from build123d import *

# Parameters (mm, degrees)
BOSS_EXTRUDE1_DEPTH = 33
SKETCH2_R           = 1
CUT_EXTRUDE1_DEPTH  = 3.5
SKETCH3_W           = 12
SKETCH3_H           = 2
BOSS_EXTRUDE2_DEPTH = 8
SKETCH4_R           = 7.5
BOSS_EXTRUDE3_DEPTH = 1.5
SKETCH5_R           = 2
BOSS_EXTRUDE4_DEPTH = 8.5


with BuildPart() as part:
    # Sketch1 → Boss-Extrude1 (new body)
    with BuildSketch(Plane.XY):
        with BuildLine():
            Line((-8.1, -10.1), (8.1, -10.1))
            ThreePointArc((8.1, -10.1), (9.514213562, -9.514213562), (10.1, -8.1))
            Line((10.1, -8.1), (10.1, 8.1))
            ThreePointArc((10.1, 8.1), (9.514213562, 9.514213562), (8.1, 10.1))
            Line((8.1, 10.1), (-8.1, 10.1))
            ThreePointArc((-8.1, 10.1), (-9.514213562, 9.514213562), (-10.1, 8.1))
            Line((-10.1, 8.1), (-10.1, -8.1))
            ThreePointArc((-10.1, -8.1), (-9.514213562, -9.514213562), (-8.1, -10.1))
        make_face()
    extrude(amount=-BOSS_EXTRUDE1_DEPTH)

    # Sketch2 → Cut-Extrude1 (cut)
    with BuildSketch(Plane.XY):
        with Locations((-8, 8)):
            Circle(SKETCH2_R)
        with Locations((8, 8)):
            Circle(SKETCH2_R)
        with Locations((8, -8)):
            Circle(SKETCH2_R)
        with Locations((-8, -8)):
            Circle(SKETCH2_R)
    extrude(amount=-CUT_EXTRUDE1_DEPTH, mode=Mode.SUBTRACT)

    # Sketch3 → Boss-Extrude2 (add)
    with BuildSketch(Plane(origin=(0, 0, -33), x_dir=(-1, 0, 0), z_dir=(0, 0, -1))):
        with Locations((0, 11.1)):
            Rectangle(SKETCH3_W, SKETCH3_H)
    extrude(amount=-BOSS_EXTRUDE2_DEPTH)

    # Sketch4 → Boss-Extrude3 (add)
    with BuildSketch(Plane.XY):
        with Locations(Location((0, 0, 0), (0, 0, 180))):
            Circle(SKETCH4_R)
    extrude(amount=BOSS_EXTRUDE3_DEPTH)

    # Sketch5 → Boss-Extrude4 (add)
    with BuildSketch(Plane.XY.offset(1.5)):
        Circle(SKETCH5_R)
    extrude(amount=BOSS_EXTRUDE4_DEPTH)


solid = part.part
Build history of the part. All positions in model axes, mm. A direction names the side the tool comes from. Round coordinates to 2 decimals unless told otherwise and drop trailing zeros. Write each loop counter-clockwise with the first axis right and the second up, starting at its lowest first coordinate (ties: lowest second). Pieces come first, ordered by that corner, then holes. Notation, with made-up numbers: (64, 81.5) - (68, 81.5) arc R19 ccw to (68, 94.5) - close; hole circle Ø5 at (87, 19.5). An arc over 180 degrees is marked (long way). One line per question, with ' | ' between items.
1. Band-saw the part on D-D, the plane x = 4.5. Write the cut outline in (y, z).
Results are:
outline: (-10.1, -33) - (12.1, -33) - (12.1, -25) - (10.1, -25) - (10.1, 0) - (6, 0) - (6, 1.5) - (-6, 1.5) - (-6, 0) - (-10.1, 0) - close
2. Band-saw the part on C-C, the plane y = 4.75. Write the cut outline in (x, z), and give its area (3 significant figures).
Results are:
outline: (-10.1, -33) - (10.1, -33) - (10.1, 0) - (5.8, 0) - (5.8, 1.5) - (-5.8, 1.5) - (-5.8, 0) - (-10.1, 0) - close | area: 684 mm^2
3. Band-saw the part on A-A, the plane z = -8.5. Write the cut outline in (x, y).
Results are:
outline: (-10.1, -8.1) arc R2 ccw to (-8.1, -10.1) - (8.1, -10.1) arc R2 ccw to (10.1, -8.1) - (10.1, 8.1) arc R2 ccw to (8.1, 10.1) - (-8.1, 10.1) arc R2 ccw to (-10.1, 8.1) - close
4. Drop flat-ended pins along their axis: pin 1 Ø0.6 at (x, y) = (-8, 8) entering from +Z; pin 2 Ø1.6 at (y, z) = (11, -28.5) entering from +X; pin 3 Ø6 at (x, z) = (-1, -15) entering from +Y. Give the stop position or say it passes through.
Results are:
pin 1: z = -3.5 | pin 2: x = 6 | pin 3: y = 10.1
5. Mould opens along Y. For faces 4 (the face through (-10.1, 0, -16)), 5 (the face through (8, 9, -2)), 6 (the face through (0, -2, 6)), 7 (the face through (-8, 9, -2)) say: released by +Y, released by -Y, zero draft, split by the parting line, or undercut.
Results are:
face 4: zero draft | face 5: undercut | face 6: split by the parting line | face 7: undercut
6. Tool access for faces 1 (the face through (0, 11, -25)), 2 (the face through (-8, -8, -3.5)), 3 (the face through (-6, 11, -29)): list every direction of +Z, -Z, +X, -X, +Y, -Y with a clear straight run to the whole face (end or side of a thin tool).
Results are:
face 1: +Z, +X, -X, +Y | face 2: +Z | face 3: +Z, -Z, -X, +Y
7. Band-saw the part on B-B, the plane x = 0. Write the cut outline in (y, z), and give its area (3 significant figures).
Results are:
outline: (-10.1, -33) - (12.1, -33) - (12.1, -25) - (10.1, -25) - (10.1, 0) - (7.5, 0) - (7.5, 1.5) - (2, 1.5) - (2, 10) - (-2, 10) - (-2, 1.5) - (-7.5, 1.5) - (-7.5, 0) - (-10.1, 0) - close | area: 739 mm^2
8. Drill centre lines: line 1 along Y through (x, z) = (8, -1.3); line 2 along X through (y, z) = (-8.5, -3); line 3 along Z through (x, y) = (5.75, 11). Where is each one in solid material? Low to high. Write a range as from..to.
Results are:
line 1: -10.1..-9, -7..7, 9..10.1 | line 2: -10.06..-8.87, -7.13..7.13, 8.87..10.06 | line 3: -33..-25
